from build123d import *

# Parameters (mm, degrees)
BOSS_EXTRUDE2_DEPTH                               = 20
CSK_FOR_3_FLAT_HEAD_MACHINE_SCREW_100_D           = 2.794
CSK_FOR_3_FLAT_HEAD_MACHINE_SCREW_100_DEPTH       = 20
CSK_FOR_3_FLAT_HEAD_MACHINE_SCREW_100_CSINK_D     = 5.0546
CSK_FOR_3_FLAT_HEAD_MACHINE_SCREW_100_CSINK_ANGLE = 100


with BuildPart() as part:
    # Sketch1 → Boss-Extrude2 (new body)
    with BuildSketch(Plane.XY):
        Polygon((0, 500.68043587), (118.58, 345.487717935), (863.58, 345.487717935), (963.71, 481.146537036), (963.71, 900.804334703), (863.58, 1036.463153804), (118.58, 1036.463153804), (0, 881.27043587), align=None)
    extrude(amount=BOSS_EXTRUDE2_DEPTH)

    # CSK for #3 Flat Head Machine Screw (100)2
    with Locations(Plane(origin=(0, 0, 0), x_dir=(-1, 0, 0), z_dir=(0, 0, -1))):
        with Locations((-950.019491684, 864.74090145), (-950.019491684, 773.32689058), (-950.019491684, 608.634912319), (-950.019491684, 517.22090145), (-905.654330921, 422.269736472), (-803.58, 360.487717935), (-633.58, 360.487717935), (-348.58, 360.487717935), (-178.58, 360.487717935), (-102.481993543, 388.446303105), (-48.296375955, 460.30671534), (-15.328698966, 580.68043587), (-15.328698966, 801.27043587), (-50.699956706, 924.831760626), (-104.885574294, 996.692172861), (-178.58, 1021.463153804), (-348.58, 1021.463153804), (-633.58, 1021.463153804), (-803.58, 1021.463153804), (-905.654330921, 959.692066427)):
            CounterSinkHole(CSK_FOR_3_FLAT_HEAD_MACHINE_SCREW_100_D / 2, CSK_FOR_3_FLAT_HEAD_MACHINE_SCREW_100_CSINK_D / 2, depth=CSK_FOR_3_FLAT_HEAD_MACHINE_SCREW_100_DEPTH, counter_sink_angle=CSK_FOR_3_FLAT_HEAD_MACHINE_SCREW_100_CSINK_ANGLE)


solid = part.part
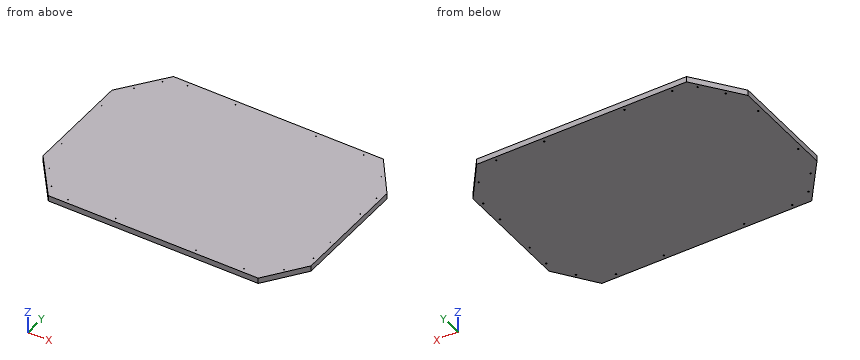
Source: CAD feature listing. Evaluate the final solid. Frame: model axes, mm. Give positions to 0.01 mm unless a question says otherwise; leave off trailing zeros. Answer as a JSON object with one key per item and string values.
Q1. Cut plane A-A, the plane z = 8. Count the separate pieces of the cut face and the enclosed holes in it, then the cut area to 3 significant figures.
Geometry check:
{"separate pieces": "1", "enclosed holes": "20", "area": "634,000 mm^2"}
Q2. Ray query, line 1 along Y through (x, z) = (803.58, 7.75); line 2 along Y through (x, z) = (880.5, 19.25); line 3 along X through (y, z) = (1004, 8.5). Return the intervals inside material, ascending.
Geometry check:
{"line 1": "y = 345.49 to 359.09, 361.88 to 1020.07, 1022.86 to 1036.46", "line 2": "y = 368.41 to 1013.54", "line 3": "x = 93.78 to 887.54"}
Q3. Contact query for flat-ended pins moving along their axis: P1, Ø3, axis at x = 178.58, y = 360.49, coming from the -Z side; P2, Ø3.5, axis at x = 102.48, y = 388.45, coming from the -Z side. Output: stop coordinate, or through.
Geometry check:
{"P1": "stops at z = 0.86", "P2": "stops at z = 0.65"}
